Autodesk Inventor part; units mm, degrees
ref_plane "РабПлоскость1" through (7, 0, -23.1662) normal (-0.7071068, -0.7071068, 0) x (0, 0, 1)
ref_plane "YZ Plane" through (0, 0, 0) normal (1, 0, 0) x (0, 1, 0)
ref_plane "XZ Plane" through (0, 0, 0) normal (0, 1, 0) x (-1, 0, 0)
sketch "Эскиз1" plane through (0, 0, 0) normal (0, 0, 1) x (1, 0, 0)
  circle A0 centre (0, 0) radius 9.5
  dimension "d0" = 19
extrude "Выдавливание1" add sketch "Эскиз1" along normal blind 4
sketch "Эскиз2" plane through (0, 0, 4) normal (0, 0, 1) x (1, 0, 0)
  circle A0 centre (0, 0) radius 7 construction
  line L0 (-7, 0) -> (7, 0) construction
  line L1 (0, 7) -> (0, -7) construction
  dimension "d3" = 14
hole "Отверстие1" at (0, 7, 4) at (0, 0, 4) at (7, 0, 4) at (-7, 0, 4) at (0, -7, 4) direction (0, 0, -1) diameter 3 end through all
ref_plane "РабПлоскость1" through (7, 0, -23.1662) normal (-0.7071068, -0.7071068, 0) x (0, 0, 1)
sketch "Эскиз4" plane through (7, 0, -23.1662) normal (-0.7071068, -0.7071068, 0) x (0, 0, 1)
  line L0 (23.1662, 3.4497) -> (23.1662, 6.4497)
  line L1 (27.1662, 6.4497) -> (27.1662, 3.4497)
  line L2 (27.1662, -4.5503) -> (27.1662, 14.4497)
  line L3 (27.1662, 4.9497) -> (23.1662, 4.9497)
  point P0 (25.1662, 4.9497)
hole "Отверстие2" at (3.5, 3.5, 2) direction (0.7071068, 0.7071068, 0) diameter 2 end through all
sketch "Эскиз5" plane through (3.5, 3.5, 2) normal (0.7071068, 0.7071068, 0) x (-0.7071068, 0.7071068, 0)
  circle A0 centre (0, 0) radius 1
  point P0 (0, -2)
hole "Отверстие3" at (3.5, 3.5, 2) direction (-0.7071068, -0.7071068, 0) diameter 2 end up to surface
thread "Резьба1"
thread "Резьба2"
thread "Резьба3"
thread "Резьба4"
thread "Резьба5"
properties part number "Планшайба D19"
Design review of the part built by this model. Coordinates are the model's own, in mm. Coordinates: 2 decimals unless noted, no trailing zeros. Write each loop counter-clockwise with the first axis right and the second up, starting at its lowest first coordinate (ties: lowest second). Pieces come first, ordered by that corner, then holes. Notation, with made-up numbers: M 75,66.5 L 131,66.5 A34 ccw 131,104.5 Z; hole C 12,8.25 d1. An arc over 180 degrees is marked long. Answer as a JSON object with one key per item and string values.
Item 1: Wall thickness on probe 1 along Y at (x, z) = (0, 2.3); probe 2 along Y at (x, z) = (7, 1.5); probe 3 along X at (y, z) = (3.75, 1.5): over which ranges is each line inside the solid? List them lowest first.
Outcome:
{"probe 1": "-9.5 to -8.5, -5.5 to -1.5, 1.5 to 5.5, 8.5 to 9.5", "probe 2": "-6.42 to -1.5, 1.5 to 5.78", "probe 3": "-8.73 to 2.53, 4.97 to 8.73"}
Item 2: Add section A-A, the plane z = 3.3. Give the boundary of the cut face in (x, y), and give its area (3 significant figures).
Outcome:
{"outline": "C 0,0 d19; hole C -7,0 d3; hole C 0,-7 d3; hole C 0,0 d3; hole C 0,7 d3; hole C 7,0 d3", "area": "248 mm²"}
Item 3: Draft analysis for pull direction Y (two halves, no side actions). For faces 1 (the cylindrical face through (4.38, 8.43, 1.97)), 2 (the cylindrical face through (-5.536, 0.325, 1.972)), 3 (the flat face through (0, -2, 4)), state which applies: pulls with the +Y half, pulls with the -Y half, needs draft (parallel to the pull), parting line crosses it, or undercut.
Outcome:
{"face 1": "parting line crosses it", "face 2": "undercut", "face 3": "needs draft"}
Item 4: Add section B-B, the plane x = -7. Give the boundary of the cut face in (y, z).
Outcome:
{"outline": "M -6.42,0 L -1.5,0 L -1.5,4 L -6.42,4 Z; M 1.5,0 L 6.42,0 L 6.42,4 L 1.5,4 Z"}
Item 5: Insertion check: pin 1 Ø2.5 at (x, y) = (0, -7) entering from -Z; pin 2 Ø1.5 at (y, z) = (5.5, 1) entering from -X. Each pin has a flat end and moves straight along its axis. Give the tip position at first contact, or say it passes through.
Outcome:
{"pin 1": "through", "pin 2": "x = -8.23"}
Item 6: Add section D-D, the plane z = 1.4. Give the boundary of the cut face in (x, y).
Outcome:
{"outline": "M 0.33,1.46 L 6.13,7.26 A9.5 ccw long 7.26,6.13 L 1.46,0.33 A1.5 cw long Z; hole C -7,0 d3; hole C 0,-7 d3; hole C 0,7 d3; hole C 7,0 d3"}
